```python
from build123d import *

# Parameters (mm, degrees)
SKETCH1_W                                      = 76.2
SKETCH1_H                                      = 177.8
BOSS_EXTRUDE1_DEPTH                            = 3.175
CSK_FOR_M3_5_FLAT_HEAD_MACHINE_SCREW1_AT_COUNT = 2
CSK_FOR_M3_5_FLAT_HEAD_MACHINE_SCREW1_AT_PITCH = 61.976
CSK_FOR_M3_5_FLAT_HEAD_MACHINE_SCREW_2_COUNT   = 2
CSK_FOR_M3_5_FLAT_HEAD_MACHINE_SCREW_2_PITCH   = 73.697214737
CSK_FOR_M3_5_FLAT_HEAD_MACHINE_SCREW_3_COUNT   = 2
CSK_FOR_M3_5_FLAT_HEAD_MACHINE_SCREW_3_PITCH   = 50.50258437
CSK_FOR_M3_5_FLAT_HEAD_MACHINE_SCREW_4_COUNT   = 2
CSK_FOR_M3_5_FLAT_HEAD_MACHINE_SCREW_4_PITCH   = 39.878
CSK_FOR_M3_5_FLAT_HEAD_MACHINE_SCREW_5_COUNT   = 2
CSK_FOR_M3_5_FLAT_HEAD_MACHINE_SCREW_5_PITCH   = 113.848594475
SKETCH7_W                                      = 11.90625
SKETCH7_H                                      = 38.1
BOSS_EXTRUDE2_DEPTH                            = 3.175
CSK_FOR_8_FLAT_HEAD_MACHINE_SCREW_2_COUNT      = 2
CSK_FOR_8_FLAT_HEAD_MACHINE_SCREW_2_PITCH      = 28.398063314
CSK_FOR_8_FLAT_HEAD_MACHINE_SCREW_3_COUNT      = 2
CSK_FOR_8_FLAT_HEAD_MACHINE_SCREW_3_PITCH      = 12.7
CSK_FOR_8_FLAT_HEAD_MACHINE_SCREW_4_COUNT      = 2
CSK_FOR_8_FLAT_HEAD_MACHINE_SCREW_4_PITCH      = 25.4
SKETCH10_W                                     = 76.2
SKETCH10_H                                     = 38.1
CUT_EXTRUDE2_DEPTH                             = 103.048594621
SKETCH11_W                                     = 49.276
SKETCH11_H                                     = 43.18
CUT_EXTRUDE3_DEPTH                             = 103.048594621
CUT_EXTRUDE4_DEPTH                             = 103.048594621
FILLET2_R                                      = 6.35
FILLET3_R                                      = 6.35


with BuildPart() as part:
    # Sketch1 → Boss-Extrude1 (new body)
    with BuildSketch(Plane(origin=(0, 0, 0), x_dir=(1, 0, 0), z_dir=(0, 1, 0))):
        Rectangle(SKETCH1_W, SKETCH1_H)
    extrude(amount=BOSS_EXTRUDE1_DEPTH)

    # Sketch5 → CSK for M3.5 Flat Head Machine Screw1 (revolve, cut)
    with BuildSketch(Plane(origin=(-30.988, 3.175, -77.978), x_dir=(0, 0, 1), z_dir=(1, 0, 0))):
        Polygon((0, 0), (0, 3.175), (1.95, 3.175), (1.95, 2.15), (4.1, 0), align=None)
    csk_for_m3_5_flat_head_machine_screw1 = revolve(axis=Axis((-30.988, 9.525, -77.978), (0, -1, 0)), mode=Mode.SUBTRACT)

    # CSK for M3.5 Flat Head Machine Screw1 at: CSK for M3.5 Flat Head Machine Screw1 ×2
    with Locations(*[(i * CSK_FOR_M3_5_FLAT_HEAD_MACHINE_SCREW1_AT_PITCH, 0, 0) for i in range(1, CSK_FOR_M3_5_FLAT_HEAD_MACHINE_SCREW1_AT_COUNT)]):
        add(csk_for_m3_5_flat_head_machine_screw1, mode=Mode.SUBTRACT)

    # CSK for M3.5 Flat Head Machine Screw 2: CSK for M3.5 Flat Head Machine Screw1 ×2
    with Locations(*[Vector(0.8409544406952484, 0, 0.5411059311030901) * (i * CSK_FOR_M3_5_FLAT_HEAD_MACHINE_SCREW_2_PITCH) for i in range(1, CSK_FOR_M3_5_FLAT_HEAD_MACHINE_SCREW_2_COUNT)]):
        add(csk_for_m3_5_flat_head_machine_screw1, mode=Mode.SUBTRACT)

    # CSK for M3.5 Flat Head Machine Screw 3: CSK for M3.5 Flat Head Machine Screw1 ×2
    with Locations(*[Vector(0.6135923613981475, 0, 0.7896229568812226) * (i * CSK_FOR_M3_5_FLAT_HEAD_MACHINE_SCREW_3_PITCH) for i in range(1, CSK_FOR_M3_5_FLAT_HEAD_MACHINE_SCREW_3_COUNT)]):
        add(csk_for_m3_5_flat_head_machine_screw1, mode=Mode.SUBTRACT)

    # CSK for M3.5 Flat Head Machine Screw 4: CSK for M3.5 Flat Head Machine Screw1 ×2
    with Locations(*[(0, 0, i * CSK_FOR_M3_5_FLAT_HEAD_MACHINE_SCREW_4_PITCH) for i in range(1, CSK_FOR_M3_5_FLAT_HEAD_MACHINE_SCREW_4_COUNT)]):
        add(csk_for_m3_5_flat_head_machine_screw1, mode=Mode.SUBTRACT)

    # CSK for M3.5 Flat Head Machine Screw 5: CSK for M3.5 Flat Head Machine Screw1 ×2
    with Locations(*[Vector(0.27218605677803737, 0, 0.9622446417079302) * (i * CSK_FOR_M3_5_FLAT_HEAD_MACHINE_SCREW_5_PITCH) for i in range(1, CSK_FOR_M3_5_FLAT_HEAD_MACHINE_SCREW_5_COUNT)]):
        add(csk_for_m3_5_flat_head_machine_screw1, mode=Mode.SUBTRACT)

    # Sketch7 → Boss-Extrude2 (add)
    with BuildSketch(Plane.XZ):
        with Locations((-44.053125, 31.75)):
            Rectangle(SKETCH7_W, SKETCH7_H)
    extrude(amount=-BOSS_EXTRUDE2_DEPTH)

    # Sketch8 → CSK for #8 Flat Head Machine Screw (100)1 (revolve, cut)
    with BuildSketch(Plane(origin=(-29.68625, 0, 44.45), x_dir=(0, 0, -1), z_dir=(1, 0, 0))):
        Polygon((0, 0), (0, 3.17505), (2.2479, 3.17505), (2.2479, 1.651767624), (4.2164, 0), align=None)
    csk_for_8_flat_head_machine_screw_100 = revolve(axis=Axis((-29.68625, -6.35, 44.45), (0, 1, 0)), mode=Mode.SUBTRACT)

    # CSK for _8 Flat Head Machine Screw _ 2: CSK for #8 Flat Head Machine Screw (100)1 ×2
    with Locations(*[Vector(-0.44721359549995776, 0, -0.8944271909999161) * (i * CSK_FOR_8_FLAT_HEAD_MACHINE_SCREW_2_PITCH) for i in range(1, CSK_FOR_8_FLAT_HEAD_MACHINE_SCREW_2_COUNT)]):
        add(csk_for_8_flat_head_machine_screw_100, mode=Mode.SUBTRACT)

    # CSK for _8 Flat Head Machine Screw _ 3: CSK for #8 Flat Head Machine Screw (100)1 ×2
    with Locations(*[(-i * CSK_FOR_8_FLAT_HEAD_MACHINE_SCREW_3_PITCH, 0, 0) for i in range(1, CSK_FOR_8_FLAT_HEAD_MACHINE_SCREW_3_COUNT)]):
        add(csk_for_8_flat_head_machine_screw_100, mode=Mode.SUBTRACT)

    # CSK for _8 Flat Head Machine Screw _ 4: CSK for #8 Flat Head Machine Screw (100)1 ×2
    with Locations(*[(0, 0, -i * CSK_FOR_8_FLAT_HEAD_MACHINE_SCREW_4_PITCH) for i in range(1, CSK_FOR_8_FLAT_HEAD_MACHINE_SCREW_4_COUNT)]):
        add(csk_for_8_flat_head_machine_screw_100, mode=Mode.SUBTRACT)

    # Sketch10 → Cut-Extrude2 (cut, through all)
    with BuildSketch(Plane.XZ):
        with Locations((0, 69.85)):
            Rectangle(SKETCH10_W, SKETCH10_H)
    extrude(amount=-CUT_EXTRUDE2_DEPTH, mode=Mode.SUBTRACT)

    # Sketch11 → Cut-Extrude3 (cut, through all)
    with BuildSketch(Plane.XZ):
        with Locations((0, -67.31)):
            Rectangle(SKETCH11_W, SKETCH11_H)
    extrude(amount=-CUT_EXTRUDE3_DEPTH, mode=Mode.SUBTRACT)

    # Sketch12 → Cut-Extrude4 (cut, through all)
    with BuildSketch(Plane.XZ):
        Polygon((7.62, 50.8), (7.62, 23.9522), (-12.7, 23.9522), (-12.7, -30.48), (38.1, -30.48), (38.1, 50.8), align=None)
    extrude(amount=-CUT_EXTRUDE4_DEPTH, mode=Mode.SUBTRACT)

    # Fillet2
    fillet2_edges = [part.edges().sort_by_distance(p)[0] for p in [
        (24.638, 1.5875, -45.72),
        (-24.638, 1.5875, -45.72),
        (38.1, 1.5875, -30.48),
        (-12.7, 1.5875, -30.48),
        (-12.7, 1.5875, 23.9522),
        (7.62, 1.5875, 23.9522),
        (-38.1, 1.5875, 12.7),
    ]]
    fillet(fillet2_edges, radius=FILLET2_R)

    # Fillet3
    fillet3_edges = [part.edges().sort_by_distance(p)[0] for p in [
        (-38.1, 1.5875, -88.9),
        (-24.638, 1.5875, -88.9),
        (24.638, 1.5875, -88.9),
        (38.1, 1.5875, -88.9),
        (7.62, 1.5875, 50.8),
    ]]
    fillet(fillet3_edges, radius=FILLET3_R)


solid = part.part
```
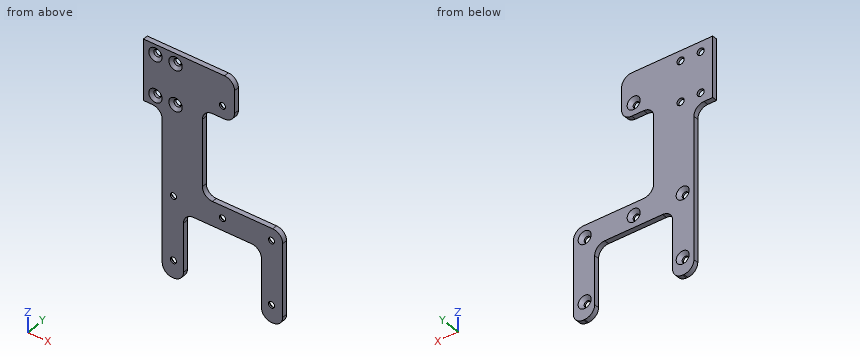
Can you work these out from the model? Positions are in its coordinate system, mm. Coordinates: 2 decimals unless noted, no trailing zeros. Write each loop counter-clockwise with the first axis right and the second up, starting at its lowest first coordinate (ties: lowest second). Pieces come first, ordered by that corner, then holes. Notation, with made-up numbers: M 69.25,32 L 89.25,32 A34 ccw 89.25,64 Z; hole C 1.25,-25 d8. An arc over 180 degrees is marked long. Write item = value, one per line. Start each with the question number.
Q1. I'm going to push flat-ended pins straight in: pin 1 (2.5 mm diameter, centred on x = -29.69, z = 19.05, fed in from +Y); pin 2 (6 mm diameter, centred on x = -42.39, z = 19.05, fed in from -Y); pin 3 (1.6 mm diameter, centred on x = -47.5, y = 1, fed in from -Z); pin 4 (1.5 mm diameter, centred on x = 2, y = 2.5, fed in from -Z). Where does each tip first touch, or does it pass through?
Q2. If I drill on L1, parallel to X at y = 0.75, z = -38.1; L2, parallel to X at y = 1.35, z = -61.5; L3, parallel to X at y = 1.5, z = 19.5, over which ranges is the centre line in solid material (lowest first)? Write a range as [from, to].
Q3. If we section it at A-A, the plane z = 19.05: Write out the boundary of the cut face in (x, y) (3 decimals).
Check sheet entries:
q1.pin_1 = through
q1.pin_2 = 1.02
q1.pin_3 = 12.7
q1.pin_4 = -45.72
q2.L1 = [-38.1, -32.94], [-29.04, -1.95], [1.95, 29.04], [32.94, 38.1]
q2.L2 = [-38.1, -24.64], [24.64, 38.1]
q2.L3 = [-50.01, -44.77], [-40, -32.07], [-27.3, -12.41]
q3.outline = M -50.006,0 L -46.603,0 L -44.634,1.652 L -44.634,3.175 L -50.006,3.175 Z; M -40.138,1.652 L -38.17,0 L -33.903,0 L -31.934,1.652 L -31.934,3.175 L -40.138,3.175 Z; M -27.438,1.652 L -25.47,0 L -12.533,0 L -12.533,3.175 L -27.438,3.175 Z
